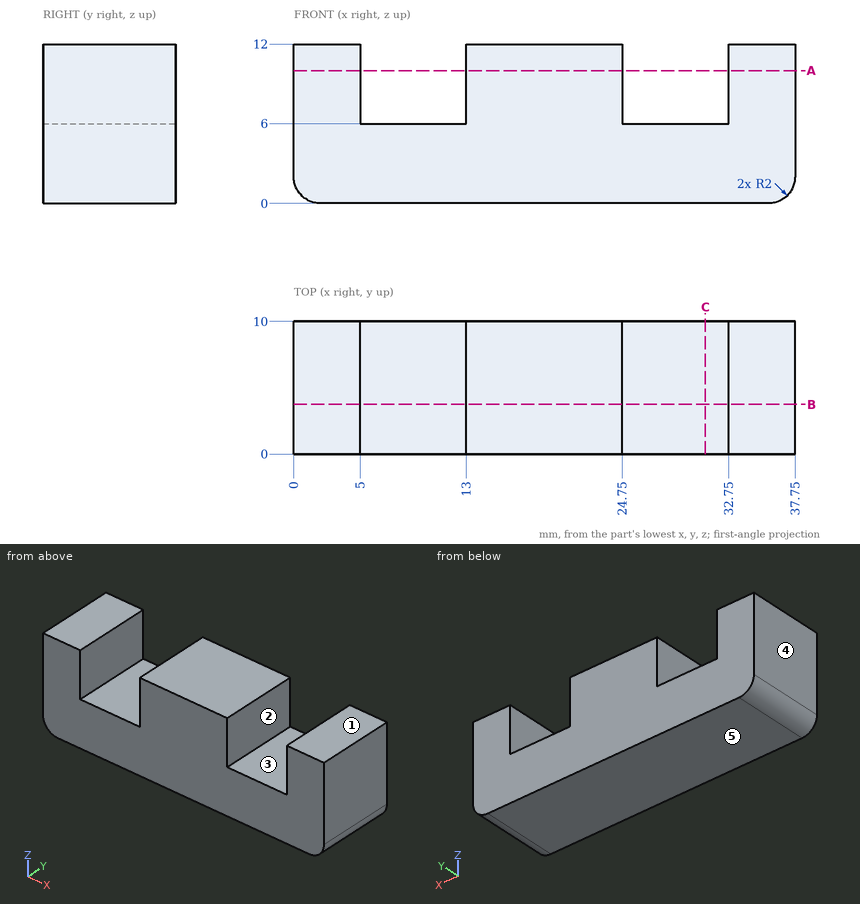
Geometry: see drawing. Coordinates: mm, zero at the bounding-box minimum. A direction names the side the tool comes from. Give positions to 0.01 mm unless a question says otherwise; leave off trailing zeros. Order: outer loops, then holes, each group sorted by start corner. A loop starts at its lowest first (then second) coordinate and runs counter-clockwise, first axis right, second up.
1. Cut plane C-C (x = 31). Return loops of the section in (y, z), and give its area (3 significant figures).
Computed:
outline: (0, 0) - (10, 0) - (10, 6) - (0, 6) - close
area: 60.0 mm2
2. Cut plane B-B (y = 3.75). Return loops of the section in (x, z), and give its area (3 significant figures).
Computed:
outline: (0, 2) arc R2 ccw to (2, 0) - (35.75, 0) arc R2 ccw to (37.75, 2) - (37.75, 12) - (32.75, 12) - (32.75, 6) - (24.75, 6) - (24.75, 12) - (13, 12) - (13, 6) - (5, 6) - (5, 12) - (0, 12) - close
area: 355 mm2
3. Line query: probe 1 along X at (y, z) = (7, 7.5); probe 2 along Z at (x, y) = (32, 5.75); probe 3 along X at (y, z) = (7.75, 0.5). Output: solid intervals per line, ascending.
Computed:
probe 1: x = 0 to 5, 13 to 24.75, 32.75 to 37.75
probe 2: z = 0 to 6
probe 3: x = 0.68 to 37.07
4. Cut plane A-A (z = 10). Return loops of the section in (x, y), and give its area (4 significant figures).
Computed:
outline: (0, 0) - (5, 0) - (5, 10) - (0, 10) - close; (13, 0) - (24.75, 0) - (24.75, 10) - (13, 10) - close; (32.75, 0) - (37.75, 0) - (37.75, 10) - (32.75, 10) - close
area: 217.5 mm2
5. Draft query along X for the marked faces 3, 4 and 5. Return one class per face: released by +X, released by -X, zero draft, split by the parting line, or undercut.
Computed:
face 3: undercut
face 4: released by -X
face 5: zero draft
6. Set-up query: the marked faces 1 and 2. Return all of +Z, -Z, +X, -X, +Y, -Y with unobstructed straight access to the full face (end or side cutting, diameter ignored); none if empty.
Computed:
face 1: +Z, +X, -X, +Y, -Y
face 2: +Z, +Y, -Y
7. Pin query (flat end, axial travel): pin 1 Ø5 at (x, y) = (8.5, 6.5) entering from +Z. Return the tip coordinate at first contact, or that it passes through.
Computed:
pin 1: stops at z = 6
